The listing builds one solid part. Answer for the finished solid, in the listing's coordinates (mm). Coordinates: 2 decimals unless noted, no trailing zeros. Loops run counter-clockwise (first coordinate to the right, second up) from the corner with the lowest first, then second, coordinate; pieces in that order, holes last. Notation, with made-up numbers: (-25, -27.5) - (-18, -27.5) arc R8 cw to (-18, -19.5) - close; hole circle Ø4 at (-38, 4). An arc over 180 degrees is marked (long way). Put each result on its own line as item: value.
```python
from build123d import *

# Parameters (mm, degrees)
F1_DEPTH = 6


with BuildPart() as f1:
    # F0 (on Front) → F1 (new body)
    with BuildSketch(Plane.XZ):
        with BuildLine():
            Line((0, 6.5), (-207.5, 6.5))
            ThreePointArc((-207.5, 6.5), (-214, 0), (-207.5, -6.5))
            Line((-207.5, -6.5), (0, -6.5))
            Line((0, -6.5), (207.5, -6.5))
            ThreePointArc((207.5, -6.5), (214, 0), (207.5, 6.5))
            Line((207.5, 6.5), (0, 6.5))
        make_face()
        with BuildLine():
            ThreePointArc((-207.5, -6), (-213.5, 0), (-207.5, 6))
            Line((-207.5, 6), (0, 6))
            Line((0, 6), (207.5, 6))
            ThreePointArc((207.5, 6), (213.5, 0), (207.5, -6))
            Line((207.5, -6), (0, -6))
            Line((0, -6), (-207.5, -6))
        make_face(mode=Mode.SUBTRACT)
    extrude(amount=F1_DEPTH)


solid = f1.part
```
1) Straight lines are drawn through the part: L1, parallel to Z at x = 80.5, y = -4.5; L2, parallel to X at y = -3, z = 0; L3, parallel to X at y = -2.9, z = 1. For each, find the intervals that lie inside material, in ascending order. Write a range as [from, to].
Found:
L1: z = [-6.5, -6], [6, 6.5]
L2: x = [-214, -213.5], [213.5, 214]
L3: x = [-213.92, -213.42], [213.42, 213.92]
2) The part is cut by section A-A (y = -5.05). Give the vertices of the cut face in (x, z), and give its area (3 significant figures).
Found:
outline: (-207.5, -6.5) - (207.5, -6.5) arc R6.5 ccw to (207.5, 6.5) - (-207.5, 6.5) arc R6.5 ccw to start; hole (-207.5, -6) - (207.5, -6) arc R6 ccw to (207.5, 6) - (-207.5, 6) arc R6 ccw to start
area: 435 mm^2
3) This flat-tipped pin is pushed along its axis until it touches: pin 1 (1.5 mm diameter, centred on y = -4.5, z = 2.5, fed in from +X). Where does it stop, or does it pass through?
Found:
pin 1: stops at x = 213.76
4) The part is cut by section C-C (x = -43). Give the vertices of the cut face in (y, z).
Found:
outline: (-6, -6.5) - (0, -6.5) - (0, -6) - (-6, -6) - close; (-6, 6) - (0, 6) - (0, 6.5) - (-6, 6.5) - close
5) The part is cut by section B-B (z = 0). Give the vertices of the cut face in (x, y), and give its area (3 significant figures).
Found:
outline: (-214, -6) - (-213.5, -6) - (-213.5, 0) - (-214, 0) - close; (213.5, -6) - (214, -6) - (214, 0) - (213.5, 0) - close
area: 6.00 mm^2
